Input: part model. Units: mm. Frame: model coordinates. A direction names the side the tool comes from. Coordinates: 2 decimals unless noted, no trailing zeros. Write each loop counter-clockwise with the first axis right and the second up, starting at its lowest first coordinate (ties: lowest second). Pieces come first, ordered by that corner, then holes. Notation, with made-up numbers: (43.25, 35) -> (81.25, 35) arc R28 cw to (81.25, 64) -> close; hole circle Ø1 at (79.25, 81.25). An arc over 180 degrees is marked (long way). Use one line per item in the form item = value. Start each with the question number.
(1) First-contact query: pin 1 (5.5 mm diameter, centred on x = 0, z = -14.5, fed in from -Y); pin 2 (1.5 mm diameter, centred on x = -0.5, y = -4.5, fed in from -Z). Flat tips, straight axial feed; report the tip coordinate or a pass-through.
(2) Set-up query: faces 1 (the face through (0, 20, -25)), 2 (the face through (3, 19.375, -17)). Return all of +Z, -Z, +X, -X, +Y, -Y with unobstructed straight access to the full face (end or side cutting, diameter ignored); none if empty.
(3) Cut plane C-C on z = -5.5. Return the cut outline in (x, y) (3 decimals).
(4) Cut plane A-A on z = -14.5. Return the cut outline in (x, y) (3 decimals), plus the area to 3 significant figures.
(5) Cut plane D-D on x = -4.5. Return the cut outline in (y, z) (3 decimals).
(6) Pull-direction query (X, two-part tool) for faces 3 (the face through (3, -21.375, -12)), 4 (the face through (-1.341, 20.361, -11.267)), 5 (the face through (12.5, 0, -1)); classes: released by +X, released by -X, zero draft, split by the parting line, or undercut.
(7) Ray query, line 1 along X through (y, z) = (19.95, -14.5); line 2 along Y through (x, z) = (-1.25, -24) (3 decimals); line 3 along Z through (x, y) = (11.75, 2.5). Return the intervals inside material, ascending.
(8) Cut plane B-B on x = 0. Return the cut outline in (y, z) (3 decimals), plus the area to 3 significant figures.
```python
from build123d import *

# Parameters (mm, degrees)
SKETCH1_W                    = 25
SKETCH1_H                    = 42.75
BASE_FLANGE2_DEPTH           = 2
EDGE_FLANGE1_STRIP_W         = 12
EDGE_FLANGE1_STRIP_H         = 2
EDGE_FLANGE1_STRIP_CUT_DEPTH = 25
EDGE_FLANGE1_DEPTH           = 25
SKETCH14_R                   = 3.5
CUT_EXTRUDE2_DEPTH           = 50.41469923


# Sheet-metal steps are written as plain solids
with BuildPart() as part:
    # Sketch1 → Base-Flange2 (new body)
    with BuildSketch(Plane.XY):
        Rectangle(SKETCH1_W, SKETCH1_H)
    extrude(amount=-BASE_FLANGE2_DEPTH)

    # Edge-Flange1 strip (across the edge) → Edge-Flange1 strip cut (cut)
    with BuildSketch(Plane(origin=(12.5, -21.375, -2), x_dir=(0, 1, 0), z_dir=(-1, 0, 0))):
        with Locations((-2, -1)):
            Rectangle(EDGE_FLANGE1_STRIP_W, EDGE_FLANGE1_STRIP_H)
    edge_flange1_strip_cut = extrude(amount=EDGE_FLANGE1_STRIP_CUT_DEPTH, mode=Mode.SUBTRACT)

    # Edge-Flange1 section (across the edge) → Edge-Flange1 (add)
    with BuildSketch(Plane(origin=(12.5, -21.375, -2), x_dir=(0, 1, 0), z_dir=(-1, 0, 0))):
        with BuildLine():
            Line((0, 2), (0, 23))
            Line((0, 23), (2, 23))
            Line((2, 23), (2, 2))
            ThreePointArc((2, 2), (2.585786438, 0.585786438), (4, 0))
            Line((4, 0), (4, -2))
            ThreePointArc((4, -2), (1.171572875, -0.828427125), (0, 2))
        make_face()
    edge_flange1 = extrude(amount=EDGE_FLANGE1_DEPTH)

    # Sketch14 → Cut-Extrude2 (cut, through all)
    with BuildSketch(Plane(origin=(0, -19.375, 0), x_dir=(1, 0, 0), z_dir=(0, 1, 0))):
        with Locations(Location((0, 14.5, 0), (0, 0, 270))):
            Circle(SKETCH14_R)
    cut_extrude2 = extrude(amount=-CUT_EXTRUDE2_DEPTH, mode=Mode.SUBTRACT)

    # Mirror1: Edge-Flange1 strip cut, Edge-Flange1, Cut-Extrude2 across plane
    add(edge_flange1_strip_cut.mirror(Plane.ZX), mode=Mode.SUBTRACT)
    add(edge_flange1.mirror(Plane.ZX))
    add(cut_extrude2.mirror(Plane.ZX), mode=Mode.SUBTRACT)


solid = part.part
```
Values:
q1.pin_1 = through
q1.pin_2 = -2
q2.face_1 = -Z, +X, -X, +Y, -Y
q2.face_2 = -Z, +X, -X
q3.outline = (-12.5, -21.375) -> (12.5, -21.375) -> (12.5, -19.375) -> (-12.5, -19.375) -> close; (-12.5, 19.375) -> (12.5, 19.375) -> (12.5, 21.375) -> (-12.5, 21.375) -> close
q4.outline = (-12.5, -21.375) -> (-3.5, -21.375) -> (-3.5, -19.375) -> (-12.5, -19.375) -> close; (-12.5, 19.375) -> (-3.5, 19.375) -> (-3.5, 21.375) -> (-12.5, 21.375) -> close; (3.5, -21.375) -> (12.5, -21.375) -> (12.5, -19.375) -> (3.5, -19.375) -> close; (3.5, 19.375) -> (12.5, 19.375) -> (12.5, 21.375) -> (3.5, 21.375) -> close
q4.area = 72.0 mm2
q5.outline = (-21.375, -25) -> (-19.375, -25) -> (-19.375, -4) arc R2 cw to (-17.375, -2) -> (17.375, -2) arc R2 cw to (19.375, -4) -> (19.375, -25) -> (21.375, -25) -> (21.375, -4) arc R4 ccw to (17.375, 0) -> (-17.375, 0) arc R4 ccw to (-21.375, -4) -> close
q6.face_3 = zero draft
q6.face_4 = undercut
q6.face_5 = released by +X
q7.line_1 = -12.5 to -3.5, 3.5 to 12.5
q7.line_2 = -21.375 to -19.375, 19.375 to 21.375
q7.line_3 = -2 to 0
q8.outline = (-21.375, -25) -> (-19.375, -25) -> (-19.375, -18) -> (-21.375, -18) -> close; (-21.375, -11) -> (-19.375, -11) -> (-19.375, -4) arc R2 cw to (-17.375, -2) -> (17.375, -2) arc R2 cw to (19.375, -4) -> (19.375, -11) -> (21.375, -11) -> (21.375, -4) arc R4 ccw to (17.375, 0) -> (-17.375, 0) arc R4 ccw to (-21.375, -4) -> close; (19.375, -25) -> (21.375, -25) -> (21.375, -18) -> (19.375, -18) -> close
q8.area = 144 mm2
